Verification items for the finished model (mm, model axes). Round coordinates to 2 decimals unless told otherwise and drop trailing zeros. Write each loop counter-clockwise with the first axis right and the second up, starting at its lowest first coordinate (ties: lowest second). Pieces come first, ordered by that corner, then holes. Notation, with made-up numbers: M -6.75,-36.5 L 43.25,-36.5 A15 ccw 43.25,-13.5 Z; hole C 21.5,64.25 d4. An arc over 180 degrees is marked long. Answer in a Markdown table with one row per item. Add a question column.
1. Go/stop test with flat-tipped pins: pin 1 Ø2.5 at (y, z) = (-65, 10) entering from -X; pin 2 Ø6 at (x, z) = (169, 6.5) entering from -Y; pin 3 Ø12 at (x, z) = (-11.5, 3.5) entering from -Y. Record where each tip stops, or that it passes through.
2. Sectioned sample at A-A on y = 4.5. Record the cut outline in (x, z) (3 decimals).
3. Material ranges on probe 1 along X at (y, z) = (-4.5, 5.5); probe 2 along Y at (x, z) = (244.5, 10) (3 decimals); probe 3 along X at (y, z) = (1, 18), recorded low to high.
4. Sectioned sample at C-C on x = 225.5. Record the cut outline in (y, z), plus the area to 3 significant figures.
5. Sectioned sample at B-B on y = -24.5. Record the cut outline in (x, z), plus the area to 3 significant figures.
```python
from build123d import *

# Parameters (mm, degrees)
SKETCH2_W           = 240
SKETCH2_H           = 10
BOSS_EXTRUDE1_DEPTH = 20
SKETCH3_R           = 2.125
CUT_EXTRUDE1_DEPTH  = 20
SKETCH4_W           = 20
SKETCH4_H           = 20
BOSS_EXTRUDE2_DEPTH = 20
SKETCH5_W           = 416
SKETCH5_H           = 20
BOSS_EXTRUDE3_DEPTH = 20
SKETCH6_W           = 10
SKETCH6_H           = 20
BOSS_EXTRUDE4_DEPTH = 95
BOSS_EXTRUDE5_REACH = 423.522
SKETCH8_W           = 68
SKETCH8_H           = 10
SKETCH8_W_2         = 240
CUT_EXTRUDE2_DEPTH  = 65
CUT_EXTRUDE3_REACH  = 425.18
SKETCH9_R           = 2.125
FILLET1_R           = 10
CUT_EXTRUDE4_REACH  = 425.18
SKETCH10_R          = 2.125


with BuildPart() as part:
    # Sketch2 → Boss-Extrude1 (new body)
    with BuildSketch(Plane.XY):
        with Locations((120, 5)):
            Rectangle(SKETCH2_W, SKETCH2_H)
    extrude(amount=BOSS_EXTRUDE1_DEPTH)

    # Sketch3 → Cut-Extrude1 (cut)
    with BuildSketch(Plane(origin=(0, 10, 0), x_dir=(1, 0, 0), z_dir=(0, 1, 0))):
        with Locations(Location((60, -10, 0), (0, 0, 270))):
            Circle(SKETCH3_R)
        with Locations(Location((120, -10, 0), (0, 0, 270))):
            Circle(SKETCH3_R)
        with Locations(Location((180, -10, 0), (0, 0, 270))):
            Circle(SKETCH3_R)
    extrude(amount=-CUT_EXTRUDE1_DEPTH, mode=Mode.SUBTRACT)

    # Sketch4 → Boss-Extrude2 (add)
    with BuildSketch(Plane(origin=(0, 10, 0), x_dir=(1, 0, 0), z_dir=(0, 1, 0))):
        with Locations((30, -10)):
            Rectangle(SKETCH4_W, SKETCH4_H)
        with Locations((210, -10)):
            Rectangle(SKETCH4_W, SKETCH4_H)
    extrude(amount=BOSS_EXTRUDE2_DEPTH)

    # Sketch5 → Boss-Extrude3 (add)
    with BuildSketch(Plane(origin=(0, 30, 0), x_dir=(1, 0, 0), z_dir=(0, 1, 0))):
        with Locations((120, -10)):
            Rectangle(SKETCH5_W, SKETCH5_H)
    extrude(amount=BOSS_EXTRUDE3_DEPTH)

    # Sketch6 → Boss-Extrude4 (add)
    with BuildSketch(Plane.XZ.offset(-30)):
        with Locations((245, 10)):
            Rectangle(SKETCH6_W, SKETCH6_H)
        with Locations((-5, 10)):
            Rectangle(SKETCH6_W, SKETCH6_H)
        with Locations((323, 10)):
            Rectangle(SKETCH6_W, SKETCH6_H)
        with Locations((-83, 10)):
            Rectangle(SKETCH6_W, SKETCH6_H)
    extrude(amount=BOSS_EXTRUDE4_DEPTH)

    # Boss-Extrude5: up to this face of the body (flat: up to its plane)
    boss_extrude5_end = Plane(part.part.faces().sort_by_distance((328, -7.5, 10))[0])
    # Sketch7 → Boss-Extrude5 (add, up to the picked face)
    with BuildSketch(Plane.ZY.offset(88), mode=Mode.PRIVATE) as boss_extrude5_sk1:
        with BuildLine():
            Line((0, -65), (20, -65))
            ThreePointArc((20, -65), (10, -75), (0, -65))
        make_face()
    boss_extrude5_tool1 = split(extrude(boss_extrude5_sk1.sketch, amount=-BOSS_EXTRUDE5_REACH, mode=Mode.PRIVATE), bisect_by=boss_extrude5_end, keep=Keep.BOTH, mode=Mode.PRIVATE)
    add(boss_extrude5_tool1.solids().sort_by(Axis((-88, -69.244132, 10), (1, 0, 0)))[0])

    # Sketch8 → Cut-Extrude2 (cut)
    with BuildSketch(Plane(origin=(0, 0, 0), x_dir=(-1, 0, 0), z_dir=(0, 0, -1))):
        with Locations((-284, -70)):
            Rectangle(SKETCH8_W, SKETCH8_H)
        with Locations((-120, -70)):
            Rectangle(SKETCH8_W_2, SKETCH8_H)
        with Locations((44, -70)):
            Rectangle(SKETCH8_W, SKETCH8_H)
    extrude(amount=-CUT_EXTRUDE2_DEPTH, mode=Mode.SUBTRACT)

    # Cut-Extrude3: up to this face of the body (flat: up to its plane)
    cut_extrude3_end = Plane(part.part.faces().sort_by_distance((328, -11.447265452, 10))[0])
    # Sketch9 → Cut-Extrude3 (cut, up to the picked face)
    with BuildSketch(Plane.ZY.offset(88), mode=Mode.PRIVATE) as cut_extrude3_sk1:
        with Locations((10, -38)):
            Circle(SKETCH9_R)
    cut_extrude3_tool1 = split(extrude(cut_extrude3_sk1.sketch, amount=-CUT_EXTRUDE3_REACH, mode=Mode.PRIVATE), bisect_by=cut_extrude3_end, keep=Keep.BOTH, mode=Mode.PRIVATE)
    add(cut_extrude3_tool1.solids().sort_by(Axis((-88, -38, 10), (1, 0, 0)))[0], mode=Mode.SUBTRACT)

    # Fillet1
    fillet1_edges = [part.edges().sort_by_distance(p)[0] for p in [
        (318, 30, 10),
        (-78, 30, 10),
        (-88, 50, 10),
        (328, 50, 10),
        (250, 30, 10),
        (-10, 30, 10),
    ]]
    fillet(fillet1_edges, radius=FILLET1_R)

    # Cut-Extrude4: up to this face of the body (flat: up to its plane)
    cut_extrude4_end = Plane(part.part.faces().sort_by_distance((-88, -16.31275275, 10))[0])
    # Sketch10 → Cut-Extrude4 (cut, up to the picked face)
    with BuildSketch(Plane(origin=(328, 0, 0), x_dir=(0, 0, -1), z_dir=(1, 0, 0)), mode=Mode.PRIVATE) as cut_extrude4_sk1:
        with Locations((-10, -65)):
            Circle(SKETCH10_R)
    cut_extrude4_tool1 = split(extrude(cut_extrude4_sk1.sketch, amount=-CUT_EXTRUDE4_REACH, mode=Mode.PRIVATE), bisect_by=cut_extrude4_end, keep=Keep.BOTH, mode=Mode.PRIVATE)
    add(cut_extrude4_tool1.solids().sort_by(Axis((328, -65, 10), (-1, 0, 0)))[0], mode=Mode.SUBTRACT)


solid = part.part
```
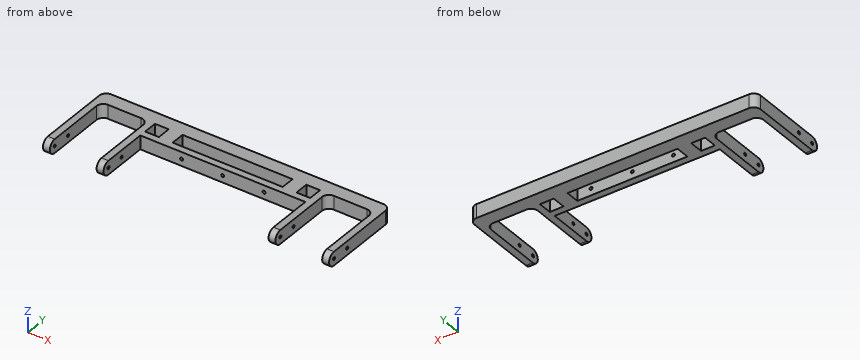
Geometry check:
| question | item | result |
|---|---|---|
| 1 | pin 1 | passes through |
| 1 | pin 2 | stops at y = 0 |
| 1 | pin 3 | stops at y = -74.98 |
| 2 | outline | M -88,0 L -78,0 L -78,20 L -88,20 Z; M -10,0 L 250,0 L 250,20 L -10,20 Z; M 318,0 L 328,0 L 328,20 L 318,20 Z; hole C 60,10 d4.25; hole C 120,10 d4.25; hole C 180,10 d4.25 |
| 3 | probe 1 | x = -88 to -78, -10 to 0, 240 to 250, 318 to 328 |
| 3 | probe 2 | y = -75 to -67.125, -62.875 to -40.125, -35.875 to 50 |
| 3 | probe 3 | x = -88 to -78, -10 to 250, 318 to 328 |
| 4 | outline | M 0,0 L 10,0 L 10,20 L 0,20 Z; M 30,0 L 50,0 L 50,20 L 30,20 Z |
| 4 | area | 600 mm2 |
| 5 | outline | M -88,0 L -78,0 L -78,20 L -88,20 Z; M -10,0 L 0,0 L 0,20 L -10,20 Z; M 240,0 L 250,0 L 250,20 L 240,20 Z; M 318,0 L 328,0 L 328,20 L 318,20 Z |
| 5 | area | 800 mm2 |
